```python
from build123d import *

# Parameters (mm, degrees)
SKETCH_1_W          = 61.5
SKETCH_1_H          = 39
EXTRUDE_1_DEPTH     = 5.5
SKETCH_2_W          = 39
SKETCH_2_H          = 3
EXTRUDE_2_DEPTH     = 0.5
SKETCH_3_W          = 62
SKETCH_3_H          = 3
EXTRUDE_3_DEPTH     = 0.5
SKETCH_5_W          = 39.5
SKETCH_5_H          = 3
EXTRUDE_4_DEPTH     = 0.5
SKETCH_6_W          = 62.5
SKETCH_6_H          = 3
EXTRUDE_5_DEPTH     = 0.5
SKETCH_7_W          = 60.5
SKETCH_7_H          = 38
CUT_EXTRUDE_1_DEPTH = 4.5
SKETCH_8_R          = 11.5
CUT_EXTRUDE_2_DEPTH = 12
SKETCH_9_R          = 2.5
EXTRUDE_7_DEPTH     = 4
SKETCH_10_R         = 1.003246397
SKETCH_10_R_2       = 1
CUT_EXTRUDE_3_DEPTH = 3


with BuildPart() as part:
    # Эскиз1 → Бобышка-Вытянуть1 (new body)
    with BuildSketch(Plane(origin=(0, 0, 0), x_dir=(1, 0, 0), z_dir=(0, 1, 0))):
        with Locations((-8.529069767, -12.848837209)):
            Rectangle(SKETCH_1_W, SKETCH_1_H)
    extrude(amount=EXTRUDE_1_DEPTH)

    # Эскиз2 → Бобышка-Вытянуть2 (add)
    with BuildSketch(Plane.ZY.offset(39.279069767)):
        with Locations((12.848837209, 4)):
            Rectangle(SKETCH_2_W, SKETCH_2_H)
    extrude(amount=EXTRUDE_2_DEPTH)

    # Эскиз3 → Бобышка-Вытянуть3 (add)
    with BuildSketch(Plane.XY.offset(32.348837209)):
        with Locations((-8.779069767, 4)):
            Rectangle(SKETCH_3_W, SKETCH_3_H)
    extrude(amount=EXTRUDE_3_DEPTH)

    # Эскиз5 → Бобышка-Вытянуть4 (add)
    with BuildSketch(Plane(origin=(22.220930233, 0, 0), x_dir=(0, 0, -1), z_dir=(1, 0, 0))):
        with Locations((-13.098837209, 4)):
            Rectangle(SKETCH_5_W, SKETCH_5_H)
    extrude(amount=EXTRUDE_4_DEPTH)

    # Эскиз6 → Бобышка-Вытянуть5 (add)
    with BuildSketch(Plane(origin=(0, 0, -6.651162791), x_dir=(-1, 0, 0), z_dir=(0, 0, -1))):
        with Locations((8.529069767, 4)):
            Rectangle(SKETCH_6_W, SKETCH_6_H)
    extrude(amount=EXTRUDE_5_DEPTH)

    # Эскиз7 → Вырез-Вытянуть1 (cut)
    with BuildSketch(Plane.XZ):
        with Locations((-8.529069767, 12.848837209)):
            Rectangle(SKETCH_7_W, SKETCH_7_H)
    extrude(amount=-CUT_EXTRUDE_1_DEPTH, mode=Mode.SUBTRACT)

    # Эскиз8 → Вырез-Вытянуть2 (cut)
    with BuildSketch(Plane(origin=(0, 5.5, 0), x_dir=(1, 0, 0), z_dir=(0, 1, 0))):
        with Locations(Location((8.220930233, -12.848837209, 0), (0, 0, 270))):
            Circle(SKETCH_8_R)
    extrude(amount=-CUT_EXTRUDE_2_DEPTH, mode=Mode.SUBTRACT)

    # Эскиз9 → Бобышка-Вытянуть7 (add)
    with BuildSketch(Plane(origin=(0, 5.5, 0), x_dir=(1, 0, 0), z_dir=(0, 1, 0))):
        with Locations(Location((8.220930233, 1.651162791, 0), (0, 0, 270))):
            Circle(SKETCH_9_R)
        with Locations(Location((8.220930233, -27.348837209, 0), (0, 0, 270))):
            Circle(SKETCH_9_R)
    extrude(amount=-EXTRUDE_7_DEPTH)

    # Эскиз10 → Вырез-Вытянуть3 (cut)
    with BuildSketch(Plane.XZ.offset(-1.5)):
        with Locations(Location((8.220930233, -1.651162791, 0), (0, 0, 270))):
            Circle(SKETCH_10_R)
        with Locations(Location((8.220930233, 27.348837209, 0), (0, 0, 270))):
            Circle(SKETCH_10_R_2)
    extrude(amount=-CUT_EXTRUDE_3_DEPTH, mode=Mode.SUBTRACT)


solid = part.part
```
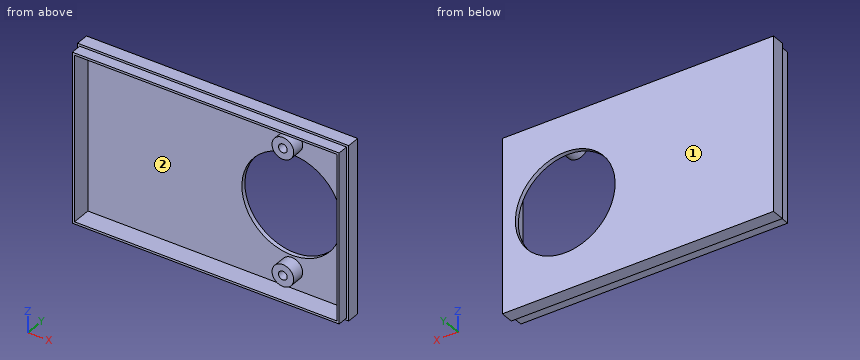
Input: part model. Units: mm. Frame: model coordinates. Face numbers are marked on the shaded views. Coordinates: 2 decimals unless noted, no trailing zeros. Loops run counter-clockwise (first coordinate to the right, second up) from the corner with the lowest first, then second, coordinate; pieces in that order, holes last. Notation, with made-up numbers: M 88.5,10.25 L 124.5,10.25 A18 ccw 124.5,40.25 Z; hole C 31,28.25 d8. An arc over 180 degrees is marked long. Use a Markdown table: item, result. Add a question column.
1) Section D-D, the plane y = 0.9. Return the cut outline in (x, z), plus the area to 3 significant figures.
2) Pin query (flat end, axial travel): P1, Ø2, axis at x = 8.5, z = -1.5, coming from the -Y side; P2, Ø20, axis at x = -20.5, z = 16, coming from the -Y side; P3, Ø0.8, axis at x = -11, y = 1.5, coming from the -Z side. Return the tip coordinate at first contact, or that it passes through.
3) Draft query along X for the marked faces 1 and 2. Return one class per face: +X half, -X half, draft (parallel to the pull), parting line (faces both ways), or undercut.
4) Line query: L1, parallel to X at y = 2, z = 17.5; L2, parallel to Z at x = -2, y = 2.1; L3, parallel to X at y = 2.6, z = 3. Output: solid intervals per line, ascending. Write a range as from..to.
5) Section B-B, the plane z = 23.5. Return the cut outline in (x, y), plus the area to 3 significant figures.
6) Section C-C, the plane x = -29. Return the cut outline in (y, z).
7) Section A-A, the plane y = 3.65. Return the cut outline in (x, z).
Answer below:
| question | item | result |
|---|---|---|
| 1 | outline | M -39.28,-6.65 L 22.22,-6.65 L 22.22,32.35 L -39.28,32.35 Z; hole M -38.78,-6.15 L 21.72,-6.15 L 21.72,31.85 L -38.78,31.85 Z |
| 1 | area | 99.5 mm2 |
| 2 | P1 | y = 1.5 |
| 2 | P2 | y = 4.5 |
| 2 | P3 | z = -6.65 |
| 3 | face 1 | draft |
| 3 | face 2 | undercut |
| 4 | L1 | -39.28..-38.78, 21.72..22.22 |
| 4 | L2 | -6.65..-6.15, 31.85..32.35 |
| 4 | L3 | -39.78..-38.78, 21.72..22.72 |
| 5 | outline | M -39.78,2.5 L -39.28,2.5 L -39.28,0 L -38.78,0 L -38.78,4.5 L 3.88,4.5 L 3.88,5.5 L -39.78,5.5 Z; M 12.56,4.5 L 21.72,4.5 L 21.72,0 L 22.22,0 L 22.22,2.5 L 22.72,2.5 L 22.72,5.5 L 12.56,5.5 Z |
| 5 | area | 60.3 mm2 |
| 6 | outline | M 0,-6.65 L 2.5,-6.65 L 2.5,-7.15 L 5.5,-7.15 L 5.5,32.85 L 2.5,32.85 L 2.5,32.35 L 0,32.35 L 0,31.85 L 4.5,31.85 L 4.5,-6.15 L 0,-6.15 Z |
| 7 | outline | M -39.78,-7.15 L 22.72,-7.15 L 22.72,32.85 L -39.78,32.85 Z; C 8.22,-1.65 d5; C 8.22,27.35 d5; hole M -38.78,-6.15 L 21.72,-6.15 L 21.72,31.85 L -38.78,31.85 Z; hole C 8.22,-1.65 d2.01; hole C 8.22,27.35 d2 |
